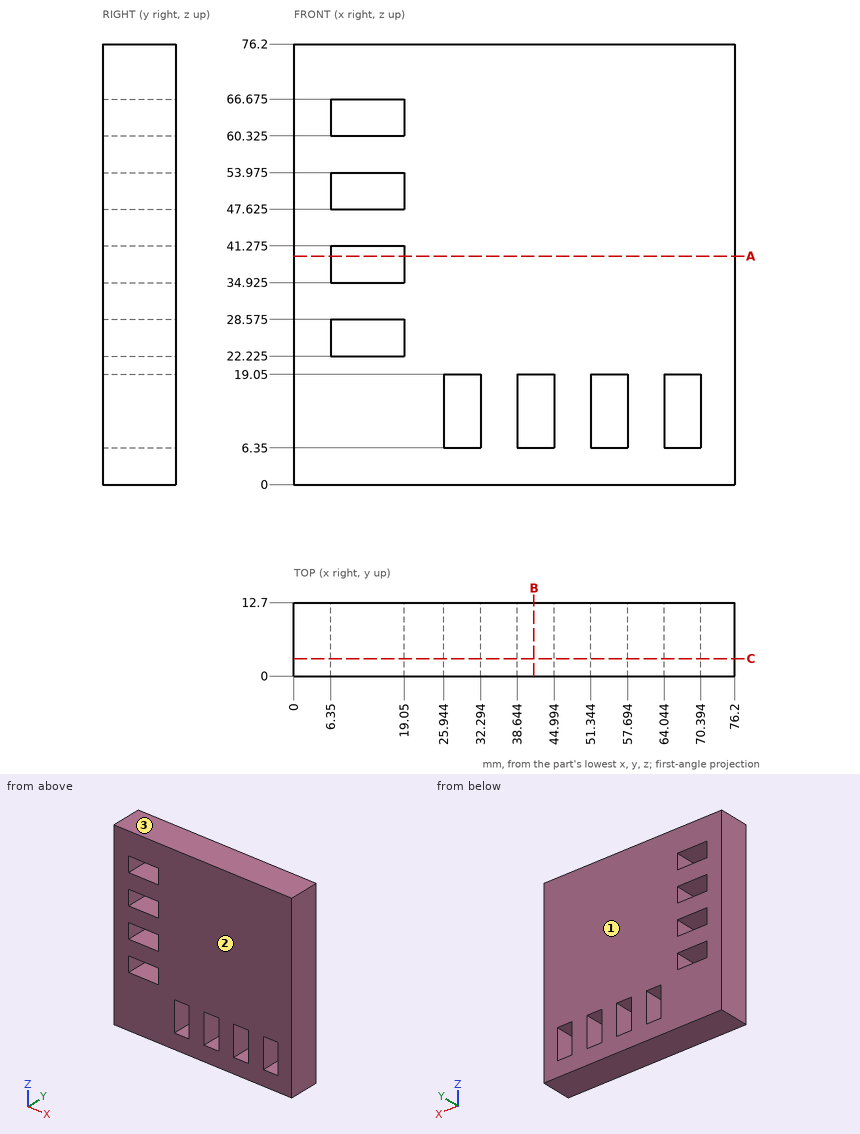
Source: three-view drawing plus pictorial views. Frame: mm from the lowest corner of the part. Round coordinates to 2 decimals unless told otherwise and drop trailing zeros. Order: outer loops, then holes, each group sorted by start corner. A loop starts at its lowest first (then second) coordinate and runs counter-clockwise, first axis right, second up. Notation, with made-up numbers: (44, 33) - (89, 33) arc R25 ccw to (89, 45) - close; hole circle Ø3 at (69, 30). An arc over 180 degrees is marked (long way). Use a Markdown table: item, result.
1. Section C-C on y = 3. State how many separate pieces and enclosed holes the cut face has, then the cut area to 3 significant figures.
Evaluation:
| item | result |
|---|---|
| separate pieces | 1 |
| enclosed holes | 8 |
| area | 5,160 mm^2 |
2. Section A-A on z = 39.5. Return the cut outline in (x, y).
Evaluation:
| item | result |
|---|---|
| outline | (0, 0) - (6.35, 0) - (6.35, 12.7) - (0, 12.7) - close; (19.05, 0) - (76.2, 0) - (76.2, 12.7) - (19.05, 12.7) - close |
3. Mould query, pull axis Y, two halves, no side actions, for the marked faces 1, 2 and 3. Classes: +Y half, -Y half, draft (parallel to the pull), parting line (faces both ways), or undercut.
Evaluation:
| item | result |
|---|---|
| face 1 | +Y half |
| face 2 | -Y half |
| face 3 | draft |
4. Section B-B on x = 41.5. Return the cut outline in (y, z).
Evaluation:
| item | result |
|---|---|
| outline | (0, 0) - (12.7, 0) - (12.7, 6.35) - (0, 6.35) - close; (0, 19.05) - (12.7, 19.05) - (12.7, 76.2) - (0, 76.2) - close |
5. Material intervals for probe 1 along X at (y, z) = (11.25, 18.5) (1 decimal); probe 2 along Z at (x, y) = (11, 1) (1 decimal); probe 3 along X at (y, z) = (7.5, 38.5), sorted ascending.
Evaluation:
| item | result |
|---|---|
| probe 1 | 0 to 25.9, 32.3 to 38.6, 45 to 51.3, 57.7 to 64, 70.4 to 76.2 |
| probe 2 | 0 to 22.2, 28.6 to 34.9, 41.3 to 47.6, 54 to 60.3, 66.7 to 76.2 |
| probe 3 | 0 to 6.35, 19.05 to 76.2 |
